```python
from build123d import *

# Parameters (mm, degrees)
BOSS_EXTRUDE1_DEPTH = 25.4
FILLET1_R           = 7.62
SKETCH2_R           = 2.921
CUT_EXTRUDE1_DEPTH  = 143.805838816
CHAMFER1_SIZE       = 1.5875
SKETCH3_R           = 3.302
CUT_EXTRUDE2_DEPTH  = 144.622345406


with BuildPart() as part:
    # Sketch1 → Boss-Extrude1 (new body)
    with BuildSketch(Plane.XY):
        Polygon((0, 0), (0, 21.59), (6.35, 21.59), (6.35, 6.35), (133.35, 6.35), (133.35, 21.59), (139.7, 21.59), (139.7, 0), align=None)
    extrude(amount=BOSS_EXTRUDE1_DEPTH)

    # Fillet1
    fillet1_edges = [part.edges().sort_by_distance(p)[0] for p in [
        (136.525, 21.59, 0),
        (136.525, 21.59, 25.4),
        (3.175, 21.59, 0),
        (3.175, 21.59, 25.4),
        (133.35, 6.35, 12.7),
        (6.35, 6.35, 12.7),
    ]]
    fillet(fillet1_edges, radius=FILLET1_R - 0.0001)  # a hair under: the kernel refuses the full size

    # Sketch2 → Cut-Extrude1 (cut, through all)
    with BuildSketch(Plane(origin=(0, 6.35, 0), x_dir=(1, 0, 0), z_dir=(0, 1, 0))):
        with Locations(Location((69.85, -12.7, 0), (0, 0, 270))):
            Circle(SKETCH2_R)
        with Locations(Location((120.65, -12.7, 0), (0, 0, 270))):
            Circle(SKETCH2_R)
        with Locations(Location((19.05, -12.7, 0), (0, 0, 270))):
            Circle(SKETCH2_R)
    extrude(amount=-CUT_EXTRUDE1_DEPTH, mode=Mode.SUBTRACT)

    # Chamfer1
    chamfer1_edges = [part.edges().sort_by_distance(p)[0] for p in [
        (139.7, 6.98505, 0),
        (133.35, 21.59, 12.7),
        (139.7, 21.59, 12.7),
        (133.35, 19.358182962, 23.168182962),
        (133.35, 19.358182962, 2.231817038),
        (0, 6.98505, 0),
        (69.85, 6.35, 0),
        (139.7, 19.358182962, 23.168182962),
        (139.7, 19.358182962, 2.231817038),
        (69.85, 6.35, 25.4),
        (0, 6.98505, 25.4),
        (0, 21.59, 12.7),
        (6.35, 21.59, 12.7),
        (0, 19.358182962, 23.168182962),
        (0, 19.358182962, 2.231817038),
        (6.35, 19.358182962, 23.168182962),
        (6.35, 19.358182962, 2.231817038),
        (131.118182962, 8.581817038, 0),
        (131.118182962, 8.581817038, 25.4),
        (8.581817038, 8.581817038, 0),
        (8.581817038, 8.581817038, 25.4),
        (139.7, 6.98505, 25.4),
    ]]
    chamfer(chamfer1_edges, length=CHAMFER1_SIZE)

    # Sketch3 → Cut-Extrude2 (cut, through all)
    with BuildSketch(Plane(origin=(139.7, 0, 0), x_dir=(0, 0, -1), z_dir=(1, 0, 0))):
        with Locations((-12.7, 12.7)):
            Circle(SKETCH3_R)
    extrude(amount=-CUT_EXTRUDE2_DEPTH, mode=Mode.SUBTRACT)


solid = part.part
```
Part model, mm, in its own coordinate system. A direction names the side the tool comes from. Round coordinates to 2 decimals unless told otherwise and drop trailing zeros. Loops run counter-clockwise (first coordinate to the right, second up) from the corner with the lowest first, then second, coordinate; pieces in that order, holes last.
Item 1: 3-axis set-ups, long thin cutter, end or side, ignore diameter. For faces 5 (the face through (8.2, 8.33, 1.14)), 6 (the face through (70.8, 0, 9.7)), 7 (the face through (6.35, 17, 13)): which of +Z, -Z, +X, -X, +Y, -Y reach the whole face in a straight line?
Item 2: Cut at C-C, the plane x = 105. Give the cut face in (y, z), then the cut area to 3 significant figures.
Item 3: Cut at A-A, the plane x = 19.05. Give the cut face in (y, z).
Item 4: Mould opens along Z. For faces 1 (the face through (136.547, 19.417, 23.109)), 2 (the face through (3, 21.59, 13)), 3 (the face through (72.313, 3.219, 14.27)), 4 (the face through (139.27, 18.59, 3.1)) say: +Z half, -Z half, draft (parallel to the pull), parting line (faces both ways), or undercut.
Item 5: Drop a flat-ended pin along its axis: P1, Ø8, axis at x = 117.5, z = 20, coming from the +Y side. Give the stop position or say it passes through.
Item 6: Cut at B-B, the plane z = 11.75. State how many separate pieces and enclosed holes the cut face has, then the cut area to 3 significant figures.
Item 7: Drill centre lines: line 1 (X direction, y = 5, z = 12.7); line 2 (X direction, y = 16, z = 18); line 3 (Y direction, x = 137.5, z = 12.7). Where is each one in solid material? Low to high.
A:
1. face 5: -Z, +Y
1. face 6: +Z, -Z, +X, -X, -Y
1. face 7: +Z, -Z, +Y
2. outline: (0, 0) - (4.76, 0) - (6.35, 1.59) - (6.35, 23.81) - (4.76, 25.4) - (0, 25.4) - close
2. area: 159 mm2
3. outline: (0, 0) - (4.76, 0) - (6.35, 1.59) - (6.35, 9.78) - (0, 9.78) - close; (0, 15.62) - (6.35, 15.62) - (6.35, 23.81) - (4.76, 25.4) - (0, 25.4) - close
4. face 1: +Z half
4. face 2: draft
4. face 3: undercut
4. face 4: -Z half
5. P1: stops at y = 6.35
6. separate pieces: 6
6. enclosed holes: 0
6. area: 911 mm2
7. line 1: x = 0 to 16.13, 21.97 to 66.93, 72.77 to 117.73, 123.57 to 139.7
7. line 2: x = 0 to 6.35, 133.35 to 139.7
7. line 3: y = 0 to 9.4, 16 to 21.59
